from build123d import *

# Parameters (mm, degrees)
SKETCH_1_W                     = 150
SKETCH_1_H                     = 15
EXTRUDE_1_DEPTH                = 20
HOLE_WIZARD_M6_1_D             = 5
HOLE_WIZARD_M6_1_2_D           = 6.6
HOLE_WIZARD_M6_1_2_CBORE_D     = 11
HOLE_WIZARD_M6_1_2_CBORE_DEPTH = 6


with BuildPart() as part:
    # 草圖1 → 伸長1 (new body)
    with BuildSketch(Plane.XY):
        Rectangle(SKETCH_1_W, SKETCH_1_H)
    extrude(amount=EXTRUDE_1_DEPTH)

    # Hole Wizard M6 _1 (through all)
    with Locations(Plane(origin=(0, 7.5, 0), x_dir=(-1, 0, 0), z_dir=(0, 1, 0))):
        with Locations((50, 10), (-50, 10)):
            Hole(HOLE_WIZARD_M6_1_D / 2)

    # Hole Wizard M6 _1 2 (through all)
    with Locations(Plane(origin=(0, 0, 0), x_dir=(-1, 0, 0), z_dir=(0, 0, -1))):
        with Locations((65, 0), (-65, 0)):
            CounterBoreHole(HOLE_WIZARD_M6_1_2_D / 2, HOLE_WIZARD_M6_1_2_CBORE_D / 2, HOLE_WIZARD_M6_1_2_CBORE_DEPTH)


solid = part.part
Can you work these out from the model? Positions are in its coordinate system, mm. A direction names the side the tool comes from. Coordinates: 2 decimals unless noted, no trailing zeros. Write each loop counter-clockwise with the first axis right and the second up, starting at its lowest first coordinate (ties: lowest second). Pieces come first, ordered by that corner, then holes. Notation, with made-up numbers: (47, -23.5) -> (67, -23.5) arc R36 cw to (67, 14.5) -> close; hole circle Ø8 at (71.5, 32). An arc over 180 degrees is marked (long way). Write each question's results on one line, items separated by ' | '. Start each with the question number.
Item 1: If we section it at A-A, the plane y = 0: Write out the boundary of the cut face in (x, z), and give its area (3 significant figures).
Item 2: If we section it at D-D, the plane x = 65: Write out the boundary of the cut face in (y, z), and give its area (3 significant figures).
Item 3: On a 3-axis mill with a long thin cutter (end or side, diameter ignored), from which of +Z, -Z, +X, -X, +Y, -Y can I reach the whole of each face in a straight line? I mean faces 1 (the flat face through (-69, 0, 6)), 2 (the cylindrical face through (-47.69, -0.1, 9.04)). Say none if no direction works.
Item 4: Please list where these lines run through material, in increasing order: probe 1 along Z at (x, y) = (-50, 2.25); probe 2 along X at (y, z) = (3, 9.25); probe 3 along Y at (x, z) = (-65.5, 1.25).
Item 5: Thinking about a two-plate mould opening in X: for faces 3 (the flat face through (-1, 0, 20)), 4 (the flat face through (75, 0, 10)), 5 (the cylindrical face through (-59.505, 0.242, 2.958)), which applies, released by +X, released by -X, zero draft, split by the parting line, or undercut?
Item 6: I'm going to push a flat-ended pin straight in: P1, Ø5.5, axis at x = -64, y = 1, coming from the -Z side. Where does the tip first touch, or does it pass through?
Item 7: If we section it at C-C, the plane x = -50: Write out the boundary of the cut face in (y, z).
Item 8: If we section it at B-B, the plane z = 10: Write out the boundary of the cut face in (x, y), and give its area (3 significant figures).
Answer block:
1) outline: (-75, 0) -> (-70.5, 0) -> (-70.5, 6) -> (-68.3, 6) -> (-68.3, 20) -> (-75, 20) -> close; (-61.7, 6) -> (-59.5, 6) -> (-59.5, 0) -> (59.5, 0) -> (59.5, 6) -> (61.7, 6) -> (61.7, 20) -> (-61.7, 20) -> close; (68.3, 6) -> (70.5, 6) -> (70.5, 0) -> (75, 0) -> (75, 20) -> (68.3, 20) -> close; hole circle Ø5 at (-50, 10); hole circle Ø5 at (50, 10) | area: 2,640 mm²
2) outline: (-7.5, 0) -> (-5.5, 0) -> (-5.5, 6) -> (-3.3, 6) -> (-3.3, 20) -> (-7.5, 20) -> close; (3.3, 6) -> (5.5, 6) -> (5.5, 0) -> (7.5, 0) -> (7.5, 20) -> (3.3, 20) -> close | area: 142 mm²
3) face 1: -Z | face 2: +Y, -Y
4) probe 1: 0 to 7.5, 12.5 to 20 | probe 2: -75 to -66.37, -63.63 to -52.38, -47.62 to 47.62, 52.38 to 63.63, 66.37 to 75 | probe 3: -7.5 to -5.48, 5.48 to 7.5
5) face 3: zero draft | face 4: released by +X | face 5: undercut
6) P1: z = 6
7) outline: (-7.5, 0) -> (7.5, 0) -> (7.5, 7.5) -> (-7.5, 7.5) -> close; (-7.5, 12.5) -> (7.5, 12.5) -> (7.5, 20) -> (-7.5, 20) -> close
8) outline: (-75, -7.5) -> (-52.5, -7.5) -> (-52.5, 7.5) -> (-75, 7.5) -> close; (-47.5, -7.5) -> (47.5, -7.5) -> (47.5, 7.5) -> (-47.5, 7.5) -> close; (52.5, -7.5) -> (75, -7.5) -> (75, 7.5) -> (52.5, 7.5) -> close; hole circle Ø6.6 at (-65, 0); hole circle Ø6.6 at (65, 0) | area: 2,030 mm²
